from build123d import *

# Parameters (mm, degrees)
ESQUISSE1_R             = 11
BOSS_EXTRU_2_DEPTH      = 4
BOSS_EXTRU_3_DEPTH      = 4
ESQUISSE6_R             = 6.5
ENL_V_MAT_EXTRU_1_DEPTH = 4
ESQUISSE7_R             = 2.5
ENL_V_MAT_EXTRU_2_DEPTH = 4
EPAISSIR3_DEPTH         = 4


# Read off the part's stored shape, not the designer's step: Boss.-Extru.3, Epaissir3
with BuildPart() as part:
    # Esquisse1 → Boss.-Extru.2 (new body)
    with BuildSketch(Plane.XY):
        Circle(ESQUISSE1_R)
    extrude(amount=BOSS_EXTRU_2_DEPTH)

    # Esquisse6 → Enlèv. mat.-Extru.1 (cut)
    with BuildSketch(Plane.XY.offset(4)):
        Circle(ESQUISSE6_R)
    extrude(amount=-ENL_V_MAT_EXTRU_1_DEPTH, mode=Mode.SUBTRACT)



with BuildPart() as body_2:
    # Boss.-Extru.3 outline → Boss.-Extru.3 (new body)
    with BuildSketch(Plane.XY):
        with BuildLine():
            ThreePointArc((26.975217648, 4.586105757), (19.99999917, -0.005763433), (26.972567207, -4.601656213))
            add(Edge.make_bspline(
                [(26.972567207, -4.601656213), (27.515164642, -4.291363801), (28.053929341, -3.966183827)],
                knots=[0.958322196, 0.958322196, 0.958322196, 1, 1, 1], degree=2))
            ThreePointArc((28.053929341, -3.966183827), (29.999998754, -0.008646725), (28.056210795, 3.95001155))
            add(Edge.make_bspline(
                [(26.975217648, 4.586105757), (27.517634871, 4.275501294), (28.056210795, 3.95001155)],
                knots=[0.958322291, 0.958322291, 0.958322291, 1, 1, 1], degree=2))
        make_face()
    extrude(amount=BOSS_EXTRU_3_DEPTH)

    # Esquisse7 → Enlèv. mat.-Extru.2 (cut)
    with BuildSketch(Plane.XY.offset(4)):
        with Locations((24.999998962, -0.007205809)):
            Circle(ESQUISSE7_R)
    extrude(amount=-ENL_V_MAT_EXTRU_2_DEPTH, mode=Mode.SUBTRACT)


with BuildPart() as part_1:
    add(part.part)

    add(body_2.part)  # Epaissir3 merges body 2
    # Epaissir3 outline → Epaissir3 (add)
    with BuildSketch(Plane.XY):
        with BuildLine():
            add(Edge.make_bspline(
                [(0, 11), (14.503070624, 11.728033327), (26.975217648, 4.586105757)],
                knots=[0, 0, 0, 0.958322291, 0.958322291, 0.958322291], degree=2))
            ThreePointArc((0, 11), (10.999999543, -0.003170596), (-0.006341192, -10.999998172))
            add(Edge.make_bspline(
                [(-0.006341192, -10.999998172), (14.496306132, -11.736391644), (26.972567207, -4.601656213)],
                knots=[0, 0, 0, 0.958322196, 0.958322196, 0.958322196], degree=2))
            ThreePointArc((26.972567207, -4.601656213), (19.99999917, -0.005763433), (26.975217648, 4.586105757))
        make_face()
    extrude(amount=EPAISSIR3_DEPTH)


solid = part_1.part
Could you check a few things on this model? Use its own coordinates, in mm. Give positions to 0.01 mm unless a question says otherwise; leave off trailing zeros. Order: outer loops, then holes, each group sorted by start corner. A loop starts at its lowest first (then second) coordinate and runs counter-clockwise, first axis right, second up.
1. I need wall thicknesses on L1, parallel to X at y = -2.25, z = 0.6; L2, parallel to Y at x = 0, z = 1.6; L3, parallel to X at y = -1.75, z = 2.05. Which ranges of each line are inside material? Lowest first, please.
Answers below:
L1: x = -10.77 to -6.1, 6.1 to 23.9, 26.1 to 29.47
L2: y = -11 to -6.5, 6.5 to 11
L3: x = -10.86 to -6.26, 6.26 to 23.21, 26.79 to 29.69
2. Suppose I cut it at C-C (z = 2.65). State how many separate pieces and enclosed holes the cut face has, plus the area to 3 significant figures.
Answers below:
separate pieces: 1
enclosed holes: 2
area: 553 mm2
3. Thinking about a two-plate mould opening in Y: for faces 1 (the flat face through (10, 0, 4)), 2 (the cylindrical face through (30, 0, 2)), 3 (the cylindrical face through (23.016, -1.528, 2.028)), which applies, +Y half, -Y half, draft (parallel to the pull), parting line (faces both ways), or undercut?
Answers below:
face 1: draft
face 2: parting line
face 3: undercut
4. Suppose I cut it at D-D (y = 1.25). Write out the boundary of the cut face in (x, z).
Answers below:
outline: (-10.93, 0) - (-6.38, 0) - (-6.38, 4) - (-10.93, 4) - close; (6.38, 0) - (22.84, 0) - (22.84, 4) - (6.38, 4) - close; (27.16, 0) - (29.84, 0) - (29.84, 4) - (27.16, 4) - close
5. Suppose I cut it at B-B (y = 3.5). Write out the boundary of the cut face in (x, z).
Answers below:
outline: (-10.43, 0) - (-5.48, 0) - (-5.48, 4) - (-10.43, 4) - close; (5.48, 0) - (28.56, 0) - (28.56, 4) - (5.48, 4) - close
6. For pin 1 (11.5 mm diameter, centred on x = 0, y = 0, fed in from +Z), with a flat end and sliding along its axis, tell me the tip position at first contact or that it passes through.
Answers below:
pin 1: passes through
7. Suppose I cut it at A-A (y = -1.25). Write out the boundary of the cut face in (x, z), plus the area to 3 significant figures.
Answers below:
outline: (-10.93, 0) - (-6.38, 0) - (-6.38, 4) - (-10.93, 4) - close; (6.38, 0) - (22.83, 0) - (22.83, 4) - (6.38, 4) - close; (27.17, 0) - (29.84, 0) - (29.84, 4) - (27.17, 4) - close
area: 94.7 mm2
